The listing builds one solid part. Answer for the finished solid, in the listing's coordinates (mm). A direction names the side the tool comes from. Give positions to 0.01 mm unless a question says otherwise; leave off trailing zeros. Write each loop counter-clockwise with the first axis right and the second up, starting at its lowest first coordinate (ties: lowest second). Pieces come first, ordered by that corner, then holes. Notation, with made-up numbers: M 89,-16.5 L 111,-16.5 A12 cw 111,4.5 Z; hole C 59.5,84.25 d9. An arc over 180 degrees is marked long. Answer as a JSON object with one key per item and string values.
```python
from build123d import *

# Parameters (mm, degrees)
CROQUIS1_R                       = 13.75
SALIENTE_EXTRUIR1_DEPTH          = 18
CROQUIS3_R                       = 8.5
SALIENTE_EXTRUIR2_DEPTH          = 4
CROQUIS4_R                       = 4.5
SALIENTE_EXTRUIR3_DEPTH          = 2
CROQUIS5_R                       = 1.5
SALIENTE_EXTRUIR4_DEPTH          = 11
CROQUIS7_R                       = 12.75
SALIENTE_EXTRUIR5_DEPTH          = 3.5
CROQUIS8_R                       = 5
SALIENTE_EXTRUIR6_DEPTH          = 2
TALADRO_DE_MARGEN_PARA_M11_D     = 3
TALADRO_DE_MARGEN_PARA_M11_DEPTH = 5


with BuildPart() as part:
    # Croquis1 → Saliente-Extruir1 (new body)
    with BuildSketch(Plane(origin=(0, 0, 0), x_dir=(1, 0, 0), z_dir=(0, 1, 0))):
        Circle(CROQUIS1_R)
    extrude(amount=SALIENTE_EXTRUIR1_DEPTH)

    # Croquis3 → Saliente-Extruir2 (add)
    with BuildSketch(Plane(origin=(0, 18, 0), x_dir=(1, 0, 0), z_dir=(0, 1, 0))):
        Circle(CROQUIS3_R)
    extrude(amount=SALIENTE_EXTRUIR2_DEPTH)

    # Croquis4 → Saliente-Extruir3 (add)
    with BuildSketch(Plane(origin=(0, 22, 0), x_dir=(1, 0, 0), z_dir=(0, 1, 0))):
        Circle(CROQUIS4_R)
    extrude(amount=SALIENTE_EXTRUIR3_DEPTH)

    # Croquis5 → Saliente-Extruir4 (add)
    with BuildSketch(Plane(origin=(0, 24, 0), x_dir=(1, 0, 0), z_dir=(0, 1, 0))):
        Circle(CROQUIS5_R)
    extrude(amount=SALIENTE_EXTRUIR4_DEPTH)

    # Croquis6 → Revolución1 (revolve)
    with BuildSketch(Plane.XY):
        Polygon((13.75, 18), (8.5, 22), (8.5, 18), align=None)
    revolve(axis=Axis((0, 18, 0), (0, -1, 0)))

    # Croquis7 → Saliente-Extruir5 (add)
    with BuildSketch(Plane.XZ):
        Circle(CROQUIS7_R)
    extrude(amount=SALIENTE_EXTRUIR5_DEPTH)

    # Croquis8 → Saliente-Extruir6 (add)
    with BuildSketch(Plane.XZ.offset(3.5)):
        with BuildLine():
            Line((7.49, 3.75), (18.76, 3.75))
            ThreePointArc((18.76, 3.75), (21.404579362, 2.654579362), (22.5, 0.01))
            Line((22.5, 0.01), (22.5, -0.01))
            ThreePointArc((22.5, -0.01), (21.404579362, -2.654579362), (18.76, -3.75))
            Line((18.76, -3.75), (7.49, -3.75))
            ThreePointArc((7.49, -3.75), (4.845420638, -4.845420638), (3.75, -7.49))
            Line((3.75, -7.49), (3.75, -18.76))
            ThreePointArc((3.75, -18.76), (2.654579362, -21.404579362), (0.01, -22.5))
            Line((0.01, -22.5), (-0.01, -22.5))
            ThreePointArc((-0.01, -22.5), (-2.654579362, -21.404579362), (-3.75, -18.76))
            Line((-3.75, -18.76), (-3.75, -7.49))
            ThreePointArc((-3.75, -7.49), (-4.845420638, -4.845420638), (-7.49, -3.75))
            Line((-7.49, -3.75), (-18.76, -3.75))
            ThreePointArc((-18.76, -3.75), (-21.404579362, -2.654579362), (-22.5, -0.01))
            Line((-22.5, -0.01), (-22.5, 0.01))
            ThreePointArc((-22.5, 0.01), (-21.404579362, 2.654579362), (-18.76, 3.75))
            Line((-18.76, 3.75), (-7.49, 3.75))
            ThreePointArc((-7.49, 3.75), (-4.845420638, 4.845420638), (-3.75, 7.49))
            Line((-3.75, 7.49), (-3.75, 18.76))
            ThreePointArc((-3.75, 18.76), (-2.654579362, 21.404579362), (-0.01, 22.5))
            Line((-0.01, 22.5), (0.01, 22.5))
            ThreePointArc((0.01, 22.5), (2.654579362, 21.404579362), (3.75, 18.76))
            Line((3.75, 18.76), (3.75, 7.49))
            ThreePointArc((3.75, 7.49), (4.845420638, 4.845420638), (7.49, 3.75))
        make_face()
        Circle(CROQUIS8_R, mode=Mode.SUBTRACT)
    extrude(amount=SALIENTE_EXTRUIR6_DEPTH)

    # Taladro de margen para M11
    with Locations(Plane(origin=(0, -5.5, 0), x_dir=(-1, 0, 0), z_dir=(0, -1, 0))):
        with Locations((0.01, 18.76), (-18.76, 0.01), (-0.01, -18.76), (18.76, -0.01)):
            Hole(TALADRO_DE_MARGEN_PARA_M11_D / 2, depth=TALADRO_DE_MARGEN_PARA_M11_DEPTH)


solid = part.part
```
1. A cutting plane is placed at C-C, the plane y = 23. Give the vertices of the cut face in (x, z).
Verdict:
{"outline": "C 0,0 d9"}
2. A cutting plane is placed at A-A, the plane x = 19.5. Give the vertices of the cut face in (y, z), plus the area to 3 significant figures.
Verdict:
{"outline": "M -5.5,-3.68 L -3.5,-3.68 L -3.5,-1.31 L -5.5,-1.31 Z; M -5.5,1.29 L -3.5,1.29 L -3.5,3.68 L -5.5,3.68 Z", "area": "9.49 mm2"}
3. For faces 4 (the cylindrical face through (-4.82, -4.49, -4.87)), 5 (the flat face through (4, 22, 4)), 6 (the flat face through (13, -4, 3.75)), 7 (the cylindrical face through (4.87, -4.49, -4.82)), determine the directions among +Z, -Z, +X, -X, +Y, -Y from which every point of the face is accessible in a straight line to the end or side of a thin tool.
Verdict:
{"face 4": "-Z, -X, -Y", "face 5": "+Y", "face 6": "+Z, +X, -Y", "face 7": "-Z, +X, -Y"}
4. The mould has two halves that part along Y. Classify faces 1 (the cylindrical face through (-2.764, -1.726, -12.447)), 2 (the cylindrical face through (-0.59, 22.99, -4.46)), 3 (the flat face through (-7, -3.5, 7)): released by +Y, released by -Y, zero draft, split by the parting line, or undercut.
Verdict:
{"face 1": "undercut", "face 2": "zero draft", "face 3": "released by -Y"}
5. Consider line 1 along Y through (x, z) = (5.5, 3); line 2 along Y through (x, z) = (20, 3); line 3 along X through (y, z) = (-4, 18). Determine where each line is inside the solid, lowest interval first.
Verdict:
{"line 1": "y = -5.5 to 22", "line 2": "y = -5.5 to -3.5", "line 3": "x = -3.75 to -1.28, 1.3 to 3.75"}
6. A cutting plane is placed at B-B, the plane y = 3.5. Give the vertices of the cut face in (x, z), plus the area to 3 significant figures.
Verdict:
{"outline": "C 0,0 d27.5", "area": "594 mm2"}
7. Flat-ended cylindrical pins translate along their axes: pin 1 (3 mm diameter, centred on x = -7, y = 8, fed in from -Z); pin 2 (1 mm diameter, centred on y = -4.5, z = 11, fed in from -X); pin 3 (2.5 mm diameter, centred on x = -0.5, z = -17.5, fed in from +Y); pin 4 (2.5 mm diameter, centred on x = 18.76, z = -0.01, fed in from +Y). Find the tip coordinate at first contact, or state that the pin passes through.
Verdict:
{"pin 1": "stops at z = -12.6", "pin 2": "stops at x = -3.75", "pin 3": "stops at y = -3.5", "pin 4": "passes through"}
